Input: part model. Units: mm. Frame: model coordinates. Face numbers are marked on the shaded views. A direction names the side the tool comes from. Coordinates: 2 decimals unless noted, no trailing zeros. Write each loop counter-clockwise with the first axis right and the second up, starting at its lowest first coordinate (ties: lowest second). Pieces come first, ordered by that corner, then holes.
1) Line query: L1, parallel to Y at x = 7, z = 2; L2, parallel to Y at x = 66, z = 9.25; L3, parallel to X at y = -18, z = 5.75. Output: solid intervals per line, ascending.
2) Section query B-B (x = 33). Output: boundary loops of the cut face in (y, z), then the cut area to 3 significant figures.
3) Draft query along Y for the marked faces 1, 2 and 3. Return one class per face: pulls with the +Y half, pulls with the -Y half, needs draft (parallel to the pull), parting line crosses it, or undercut.
4) Set-up query: the marked faces 4 and 5. Return all of +Z, -Z, +X, -X, +Y, -Y with unobstructed straight access to the full face (end or side cutting, diameter ignored); none if empty.
5) Section query A-A (y = -6). Output: boundary loops of the cut face in (x, z), then the cut area to 3 significant figures.
6) Pin query (flat end, axial travel): pin 1 Ø3 at (y, z) = (-37, 5.5) entering from -X; pin 2 Ø5 at (y, z) = (-27, 6.5) entering from -X; pin 3 Ø8 at (y, z) = (-39.5, 6.5) entering from -X. Return the tip coordinate at first contact, or that it passes through.
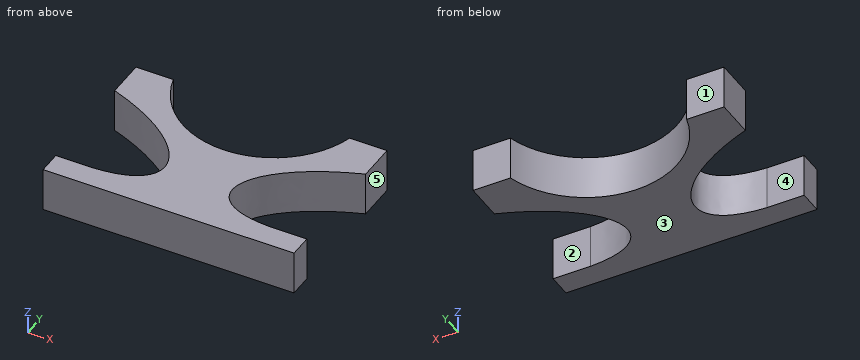
from build123d import *

# Parameters (mm, degrees)
SKETCH_1_W          = 86
SKETCH_1_H          = 58
EXTRUDE_1_DEPTH     = 15
SKETCH_3_R          = 31.2
CUT_EXTRUDE_1_DEPTH = 32
CUT_EXTRUDE_2_DEPTH = 32


with BuildPart() as part:
    # Эскиз1 → Вытянуть1 (new body)
    with BuildSketch(Plane.XY):
        with Locations((43, -29)):
            Rectangle(SKETCH_1_W, SKETCH_1_H)
    extrude(amount=EXTRUDE_1_DEPTH)

    # Эскиз3 → Вырез-Вытянуть1 (cut)
    with BuildSketch(Plane.XY):
        with Locations((43, 7.896260015)):
            Circle(SKETCH_3_R)
    extrude(amount=CUT_EXTRUDE_1_DEPTH, mode=Mode.SUBTRACT)

    # Эскиз6 → Вытянуть2 (cut)
    with BuildSketch(Plane.XY.offset(15)):
        with BuildLine():
            Line((0, -50), (12.775606869, -50))
            add(Edge.make_bspline(
                [(0, -13.292808008), (34.657854921, -25.467090291), (43.133531195, -48.731284944), (12.775606869, -50)],
                knots=[0, 0, 0, 0, 0.936580046, 0.936580046, 0.936580046, 0.936580046], degree=3))
            Line((0, -13.292808008), (-6.736902967, -13.292808008))
            Line((-6.736902967, -13.292808008), (-6.736902967, -50))
            Line((-6.736902967, -50), (0, -50))
        make_face()
        with BuildLine():
            Line((86, -50), (73.224393131, -50))
            add(Edge.make_bspline(
                [(86, -13.292808008), (51.342145079, -25.467090291), (42.866468805, -48.731284944), (73.224393131, -50)],
                knots=[0, 0, 0, 0, 0.936580046, 0.936580046, 0.936580046, 0.936580046], degree=3))
            Line((86, -13.292808008), (92.736902967, -13.292808008))
            Line((92.736902967, -13.292808008), (92.736902967, -50))
            Line((92.736902967, -50), (86, -50))
        make_face()
    extrude(amount=-CUT_EXTRUDE_2_DEPTH, mode=Mode.SUBTRACT)


solid = part.part
Answer:
1. L1: y = -58 to -50, -16.05 to 0
1. L2: y = -58 to -49.16, -23.33 to -13.19
1. L3: x = 11.13 to 25.6, 60.4 to 74.87
2. outline: (-58, 0) - (-21.66, 0) - (-21.66, 15) - (-58, 15) - close
2. area: 545 mm2
3. face 1: pulls with the +Y half
3. face 2: undercut
3. face 3: needs draft
4. face 4: +Z, -Z, -X
4. face 5: +Z, -Z, +X, +Y, -Y
5. outline: (0, 0) - (15.07, 0) - (15.07, 15) - (0, 15) - close; (70.93, 0) - (86, 0) - (86, 15) - (70.93, 15) - close
5. area: 452 mm2
6. pin 1: stops at x = 30.68
6. pin 2: stops at x = 21.56
6. pin 3: stops at x = 30.17
